Autodesk Inventor part; units mm, degrees
ref_plane "YZ Plane" through (0, 0, 0) normal (1, 0, 0) x (0, 1, 0)
ref_plane "XZ Plane" through (0, 0, 0) normal (0, 1, 0) x (-1, 0, 0)
ref_plane "XY Plane" through (0, 0, 0) normal (0, 0, 1) x (1, 0, 0)
sketch "Sketch1" plane through (0, 0, 0) normal (0, 1, 0) x (-1, 0, 0)
  circle A0 centre (0, 0) radius 10.5
  dimension "d0" = 21
extrude "Extrusion1" add sketch "Sketch1" along normal blind 1.9
sketch "Sketch2" plane through (0, 1.9, 0) normal (0, 1, 0) x (1, 0, 0)
  circle A0 centre (0, 0) radius 4.4
  dimension "d3" = 8.8
extrude "Extrusion2" add sketch "Sketch2" along normal blind 3.5
sketch "Sketch3" plane through (0, 5.4, 0) normal (0, 1, 0) x (1, 0, 0)
  circle A0 centre (0, 0) radius 1.25
  dimension "d6" = 2.5
extrude "Extrusion3" cut sketch "Sketch3" against normal through all
sketch "Sketch4" plane through (0, 0, 0) normal (0, -1, 0) x (1, 0, 0)
  circle A0 centre (7.5, 0) radius 0.95
  circle A1 centre (7.5, -3.4) radius 0.95
  circle A2 centre (7.5, 3.4) radius 0.95
  point P0 (0, 0)
  dimension "d9" = 1.9
  dimension "d10" = 7.5
  dimension "d11" = 1.9
  dimension "d12" = 3.4
  dimension "d13" = 7.5
  dimension "d14" = 1.9
  dimension "d15" = 3.4
  dimension "d16" = 7.5
extrude "Extrusion4" cut sketch "Sketch4" against normal through all
pattern_circular "Circular Pattern1" count 4 over 360 about axis through (0, -10, 0) along (0, 1, 0) of "Extrusion4"
equation "\"d15\" = d12"
properties part number "horn"
Check sheet for the modelled part. Datum: model origin and axes. Units: mm. A direction names the side the tool comes from. Give positions to 0.01 mm unless a question says otherwise; leave off trailing zeros. Write each loop counter-clockwise with the first axis right and the second up, starting at its lowest first coordinate (ties: lowest second). Pieces come first, ordered by that corner, then holes.
Item 1: Cross-section at B-B (x = 7.5). Enter the section's corners in (y, z).
Item 2: Cross-section at D-D (x = 2.75). Enter the section's corners in (y, z), and give its area (3 significant figures).
Item 3: Gauge pin test, flat ends, axial feed: pin 1 (3 mm diameter, centred on x = 0, z = 0, fed in from +Y); pin 2 (1.1 mm diameter, centred on x = 7.5, z = 3.4, fed in from -Y); pin 3 (2.5 mm diameter, centred on x = 3.4, z = 7.5, fed in from +Y). Record the tip position at first contact, or that the pin passes through.
Item 4: Cross-section at C-C (z = -3.4). Enter the section's corners in (x, y).
Item 5: Draft check along X on faces 3 (the face through (3.36, 0.94, 6.55)), 4 (the face through (-10, 0.9, -3.2)), 5 (the face through (1, 5.4, 1)). Enter one of: released by +X, released by -X, zero draft, split by the parting line, or undercut.
Item 6: Cross-section at A-A (z = 0). Enter the section's corners in (x, y), and give its area (3 significant figures).
Item 7: Access from +Z, -Z, +X, -X, +Y, -Y to the whole of each face (thin tool, end or side, straight path). Record for faces 1 (the face through (4.197, 3.626, 1.322)), 2 (the face through (-6.55, 0.94, 3.36)).
Item 8: Scan lines: L1, parallel to X at y = 0.5, z = -4; L2, parallel to X at y = 0.95, z = -7.5; L3, parallel to X at y = 3.7, z = 0. Record each from-to range of solid material in increasing order.
Report:
1. outline: (0, -7.35) - (1.9, -7.35) - (1.9, -4.35) - (0, -4.35) - close; (0, -2.45) - (1.9, -2.45) - (1.9, -0.95) - (0, -0.95) - close; (0, 0.95) - (1.9, 0.95) - (1.9, 2.45) - (0, 2.45) - close; (0, 4.35) - (1.9, 4.35) - (1.9, 7.35) - (0, 7.35) - close
2. outline: (0, -10.13) - (1.9, -10.13) - (1.9, -8.19) - (0, -8.19) - close; (0, -6.81) - (1.9, -6.81) - (1.9, -3.43) - (5.4, -3.43) - (5.4, 3.43) - (1.9, 3.43) - (1.9, 6.81) - (0, 6.81) - close; (0, 8.19) - (1.9, 8.19) - (1.9, 10.13) - (0, 10.13) - close
2. area: 57.3 mm2
3. pin 1: stops at y = 5.4
3. pin 2: passes through
3. pin 3: stops at y = 1.9
4. outline: (-9.93, 0) - (-8.45, 0) - (-8.45, 1.9) - (-9.93, 1.9) - close; (-6.55, 0) - (6.55, 0) - (6.55, 1.9) - (2.79, 1.9) - (2.79, 5.4) - (-2.79, 5.4) - (-2.79, 1.9) - (-6.55, 1.9) - close; (8.45, 0) - (9.93, 0) - (9.93, 1.9) - (8.45, 1.9) - close
5. face 3: undercut
5. face 4: split by the parting line
5. face 5: zero draft
6. outline: (-10.5, 0) - (-8.45, 0) - (-8.45, 1.9) - (-10.5, 1.9) - close; (-6.55, 0) - (-1.25, 0) - (-1.25, 5.4) - (-4.4, 5.4) - (-4.4, 1.9) - (-6.55, 1.9) - close; (1.25, 0) - (6.55, 0) - (6.55, 1.9) - (4.4, 1.9) - (4.4, 5.4) - (1.25, 5.4) - close; (8.45, 0) - (10.5, 0) - (10.5, 1.9) - (8.45, 1.9) - close
6. area: 50.0 mm2
7. face 1: +Y
7. face 2: +Y, -Y
8. L1: x = -9.71 to -8.24, -6.76 to 6.76, 8.24 to 9.71
8. L2: x = -7.35 to -4.35, -2.45 to -0.95, 0.95 to 2.45, 4.35 to 7.35
8. L3: x = -4.4 to -1.25, 1.25 to 4.4
